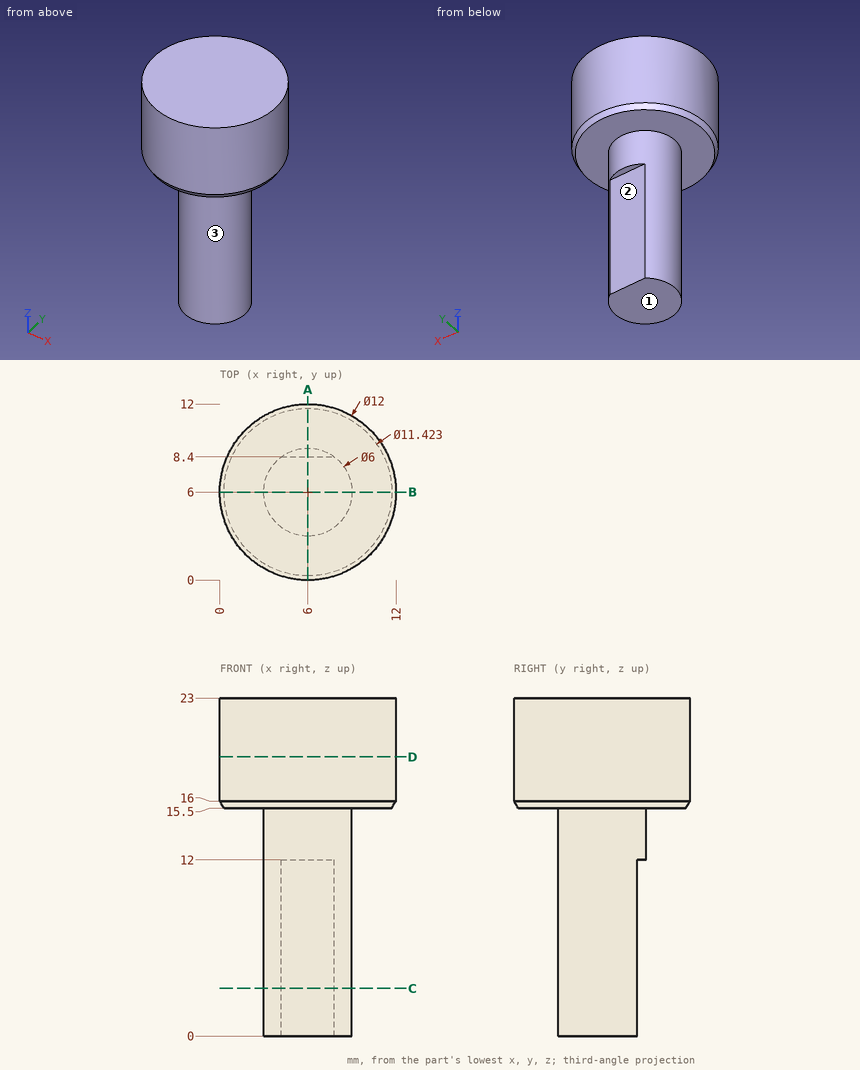
Can you work these out from the drawing? Everything is in mm from the part's minimum corner. A direction names the side the tool comes from. Round coordinates to 2 decimals unless told otherwise and drop trailing zeros. Loops run counter-clockwise (first coordinate to the right, second up) from the corner with the lowest first, then second, coordinate; pieces in that order, holes last. Notation, with made-up numbers: (33.25, 53.5) - (53.25, 53.5) arc R8 ccw to (53.25, 67.5) - close; hole circle Ø1 at (5, 57.25). An arc over 180 degrees is marked (long way). Answer in a Markdown table with one row per item. Add a question column.
Q1. I need wall thicknesses on L1, parallel to Z at x = 8, y = 10.5; L2, parallel to X at y = 5.75, z = 12; L3, parallel to X at y = 5.25, z = 11.5 (1 decimal). Which ranges of each line are inside material? Lowest first, please.
Q2. I want a section at C-C on z = 3.25. List the corners of the cut face in (x, y) for me, and give its area (3 significant figures).
Q3. I want a section at B-B on y = 6. List the corners of the cut face in (x, z) for me.
Q4. Which directions (+Z, -Z, +X, -X, +Y, -Y) give clear straight access to the entire face, cutting with the end or side of a thin tool? Please do the marked faces 1, 2 and 3.
Q5. For pin 1 Ø3 at (y, z) = (9.5, 12) entering from +X (1 decimal); pin 2 Ø3 at (y, z) = (8.5, 14.5) entering from +X; pin 3 Ø3 at (x, z) = (6, 7) entering from +Y, each with a flat end and sliding along its axis, tell me the tip position at first contact or that it passes through.
Q6. I want a section at D-D on z = 19. List the corners of the cut face in (x, y) for me.
Q7. I want a section at A-A on x = 6. List the corners of the cut face in (y, z) for me.
A:
| question | item | result |
|---|---|---|
| 1 | L1 | 15.5 to 23 |
| 1 | L2 | 3.01 to 8.99 |
| 1 | L3 | 3.1 to 8.9 |
| 2 | outline | (4.2, 8.4) arc R3 ccw (long way) to (7.8, 8.4) - close |
| 2 | area | 26.8 mm^2 |
| 3 | outline | (0, 16) - (0.29, 15.5) - (3, 15.5) - (3, 0) - (9, 0) - (9, 15.5) - (11.71, 15.5) - (12, 16) - (12, 23) - (0, 23) - close |
| 4 | face 1 | -Z, +X, -X, +Y, -Y |
| 4 | face 2 | -Z, +X, -X, +Y |
| 4 | face 3 | -Z |
| 5 | pin 1 | x = 8.2 |
| 5 | pin 2 | x = 11.62 |
| 5 | pin 3 | y = 8.4 |
| 6 | outline | circle Ø12 at (6, 6) |
| 7 | outline | (0, 16) - (0.29, 15.5) - (3, 15.5) - (3, 0) - (8.4, 0) - (8.4, 12) - (9, 12) - (9, 15.5) - (11.71, 15.5) - (12, 16) - (12, 23) - (0, 23) - close |
